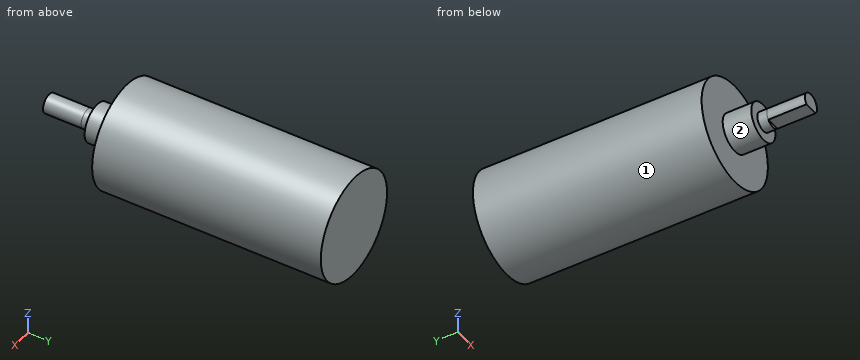
from build123d import *

# Parameters (mm, degrees)
BOSS_EXTRUDE1_DEPTH = 8
SKETCH2_R           = 2
BOSS_EXTRUDE2_DEPTH = 2
SKETCH3_R           = 4
BOSS_EXTRUDE3_DEPTH = 6
SKETCH4_R           = 11
BOSS_EXTRUDE4_DEPTH = 48


with BuildPart() as part:
    # Sketch1 → Boss-Extrude1 (new body)
    with BuildSketch(Plane(origin=(0, 0, 0), x_dir=(1, 0, 0), z_dir=(0, 1, 0))):
        with BuildLine():
            Line((-1.5, 1.322875656), (1.5, 1.322875656))
            ThreePointArc((1.5, 1.322875656), (0, -2), (-1.5, 1.322875656))
        make_face()
    extrude(amount=BOSS_EXTRUDE1_DEPTH)

    # Sketch2 → Boss-Extrude2 (add)
    with BuildSketch(Plane(origin=(0, 8, 0), x_dir=(1, 0, 0), z_dir=(0, 1, 0))):
        Circle(SKETCH2_R)
    extrude(amount=BOSS_EXTRUDE2_DEPTH)

    # Sketch3 → Boss-Extrude3 (add)
    with BuildSketch(Plane(origin=(0, 10, 0), x_dir=(1, 0, 0), z_dir=(0, 1, 0))):
        Circle(SKETCH3_R)
    extrude(amount=BOSS_EXTRUDE3_DEPTH)

    # Sketch4 → Boss-Extrude4 (add)
    with BuildSketch(Plane(origin=(0, 16, 0), x_dir=(1, 0, 0), z_dir=(0, 1, 0))):
        Circle(SKETCH4_R)
    extrude(amount=BOSS_EXTRUDE4_DEPTH)


solid = part.part
Verification items for the finished model (mm, model axes). Face numbers are marked on the shaded views. A direction names the side the tool comes from. Coordinates: 2 decimals unless noted, no trailing zeros. Write each loop counter-clockwise with the first axis right and the second up, starting at its lowest first coordinate (ties: lowest second). Pieces come first, ordered by that corner, then holes. Notation, with made-up numbers: (60.25, 55) - (90.25, 55) arc R16 cw to (90.25, 61) - close; hole circle Ø3 at (22.5, 57). An arc over 180 degrees is marked (long way). Answer as a JSON object with one key per item and string values.
(1) Gauge pin test, flat ends, axial feed: pin 1 Ø2 at (y, z) = (36.5, -4.5) entering from -X; pin 2 Ø1.5 at (y, z) = (18.5, 8) entering from +X; pin 3 Ø1 at (x, z) = (7.5, 2.5) entering from -Y. Record the tip position at first contact, or that the pin passes through.
Report:
{"pin 1": "x = -10.43", "pin 2": "x = 8.27", "pin 3": "y = 16"}
(2) Thickness scan on line 1 along Y through (x, z) = (2.25, -3); line 2 along Y through (x, z) = (-4, 4.75); line 3 along X through (y, z) = (60.5, -6.25). Record the ranges inside material, lowest first.
Report:
{"line 1": "10 to 64", "line 2": "16 to 64", "line 3": "-9.05 to 9.05"}
(3) Cross-section at C-C on y = 52.5. Record the cut outline in (x, z).
Report:
{"outline": "circle Ø22 at (0, 0)"}
(4) Tool access check on the marked faces 1 and 2. Record the directions out of +Z, -Z, +X, -X, +Y, -Y that give a thin tool (end or side, any length) a straight path to the whole face; none if there is none.
Report:
{"face 1": "+Y, -Y", "face 2": "-Y"}
(5) Cross-section at A-A on z = 0. Record the cut outline in (x, y).
Report:
{"outline": "(-11, 16) - (-4, 16) - (-4, 10) - (-2, 10) - (-2, 0) - (2, 0) - (2, 10) - (4, 10) - (4, 16) - (11, 16) - (11, 64) - (-11, 64) - close"}
(6) Cross-section at D-D on x = -2.75. Record the cut outline in (y, z), plus the area to 3 significant figures.
Report:
{"outline": "(10, -2.9) - (16, -2.9) - (16, -10.65) - (64, -10.65) - (64, 10.65) - (16, 10.65) - (16, 2.9) - (10, 2.9) - close", "area": "1,060 mm^2"}
(7) Cross-section at B-B on x = 0. Record the cut outline in (y, z).
Report:
{"outline": "(0, -1.32) - (8, -1.32) - (8, -2) - (10, -2) - (10, -4) - (16, -4) - (16, -11) - (64, -11) - (64, 11) - (16, 11) - (16, 4) - (10, 4) - (10, 2) - (0, 2) - close"}
